Input: part model. Units: mm. Frame: model coordinates. A direction names the side the tool comes from. Round coordinates to 2 decimals unless told otherwise and drop trailing zeros. Loops run counter-clockwise (first coordinate to the right, second up) from the corner with the lowest first, then second, coordinate; pieces in that order, holes last. Notation, with made-up numbers: (55.5, -13) - (95.5, -13) arc R13 ccw to (95.5, -1) - close; hole circle Ø3 at (-25.5, 26). An arc over 180 degrees is marked (long way). Use CSV: the item, a comma, the result in double quotes. Start each with the question number.
1. Cut plane A-A (x = 0). Return loops of the section in (y, z), and give its area (3 significant figures).
2. Pull-direction query (X, two-part tool) for faces 1 (the flat face through (0, 2.2, -4)), 2 (the cylindrical face through (-0.63, 0.51, -6.68)), 3 (the flat face through (0, 0, -6)); classes: +X half, -X half, draft (parallel to the pull), parting line (faces both ways), or undercut.
3. Pin query (flat end, axial travel): P1, Ø1.1, axis at x = 0.5, z = -3.5, coming from the -Y side; P2, Ø1, axis at y = 2.5, z = -6, coming from the -X side; P3, Ø2, axis at y = 2.5, z = -5.5, coming from the +X side. Return the tip coordinate at first contact, or that it passes through.
4. Cut plane D-D (x = 2.4). Return loops of the section in (y, z), and give its area (3 significant figures).
5. Access query for faces 4 (the flat face through (0, 3.6, -4)), 5 (the cylindrical face through (-0.3, 1.91, -1.57)), 6 (the cylindrical face through (1.717, 1.085, -3.309)). Directions: +Z, -Z, +X, -X, +Y, -Y. A direction counts if a zero-diameter tool reaches every point of the face in a straight line with its end or side. Return the directions, or none.
6. Cut plane B-B (y = 1.3). Return loops of the section in (x, z).
7. Cut plane C-C (y = 2.9). Return loops of the section in (x, z).
8. Material intervals for probe 1 along Z at (x, y) = (0, 1.1); probe 2 along Y at (x, z) = (-0.8, -5.1); probe 3 along X at (y, z) = (1.35, -5.3), sorted ascending. Write a range as from..to.
```python
from build123d import *

# Parameters (mm, degrees)
SKETCH_5_R          = 1.8
CUT_EXTRUDE_1_DEPTH = 2.2


with BuildPart() as part:
    # 草图2 → 旋转1 (revolve)
    with BuildSketch(Plane.XY.offset(-3.85000283)):
        with BuildLine():
            Line((1.5, 3.6), (0, 3.6))
            Line((0, 3.6), (0, 0))
            Line((0, 0), (2.9, 0))
            Line((2.9, 0), (2.9, 1))
            Line((2.9, 1), (2.3, 1))
            Line((2.3, 1), (2.3, 2.8))
            ThreePointArc((2.3, 2.8), (2.065685425, 3.365685425), (1.5, 3.6))
        make_face()
    revolve(axis=Axis((0, 3.6, -3.85000283), (0, -1, 0)))

    # 草图5 → 切除-拉伸1 (cut)
    with BuildSketch(Plane.XZ):
        with Locations((0, -3.85000283)):
            Circle(SKETCH_5_R)
    extrude(amount=-CUT_EXTRUDE_1_DEPTH, mode=Mode.SUBTRACT)


solid = part.part
```
Established:
1,outline,"(0, -6.75) - (1, -6.75) - (1, -6.15) - (2.8, -6.15) arc R0.8 ccw to (3.6, -5.35) - (3.6, -2.35) arc R0.8 ccw to (2.8, -1.55) - (1, -1.55) - (1, -0.95) - (0, -0.95) - (0, -2.05) - (2.2, -2.05) - (2.2, -5.65) - (0, -5.65) - close"
1,area,"9.57 mm2"
2,face 1,"undercut"
2,face 2,"parting line"
2,face 3,"draft"
3,P1,"stops at y = 2.2"
3,P2,"stops at x = -1.6"
3,P3,"stops at x = 2.21"
4,outline,"(0, -5.48) - (1, -5.48) - (1, -2.22) - (0, -2.22) - close"
4,area,"3.26 mm2"
5,face 4,"+Z, -Z, +X, -X, +Y"
5,face 5,"+Y"
5,face 6,"-Y"
6,outline,"circle Ø4.6 at (0, -3.85); hole circle Ø3.6 at (0, -3.85)"
7,outline,"circle Ø4.59 at (0, -3.85)"
8,probe 1,"z = -6.15..-5.65, -2.05..-1.55"
8,probe 2,"y = 2.2..3.6"
8,probe 3,"x = -1.79..-1.07, 1.07..1.79"
